Design review of the part built by this model. Coordinates are the model's own, in mm. A direction names the side the tool comes from. Coordinates: 2 decimals unless noted, no trailing zeros. Order: outer loops, then holes, each group sorted by start corner. A loop starts at its lowest first (then second) coordinate and runs counter-clockwise, first axis right, second up. Notation, with made-up numbers: (52, 64.5) - (59, 64.5) arc R12 ccw to (59, 78.5) - close; hole circle Ø10 at (-14, -39). An arc over 180 degrees is marked (long way). Write each question's results on one line, items separated by ' | '. Start each with the question number.
```python
from build123d import *

# Parameters (mm, degrees)
SKETCH1_W                                       = 146
SKETCH1_H                                       = 85
BOSS_EXTRUDE1_DEPTH                             = 15
SHELL1_T                                        = -5
SKETCH2_W                                       = 5
SKETCH2_H                                       = 75
CUT_EXTRUDE1_DEPTH                              = 10
BOSS_EXTRUDE2_DEPTH                             = 10
CSK_FOR_M3_FLAT_HEAD_MACHINE_SCREW1_D           = 3.4
CSK_FOR_M3_FLAT_HEAD_MACHINE_SCREW1_DEPTH       = 10
CSK_FOR_M3_FLAT_HEAD_MACHINE_SCREW1_CSINK_D     = 6.3
CSK_FOR_M3_FLAT_HEAD_MACHINE_SCREW1_CSINK_ANGLE = 90
CSK_FOR_M3_FLAT_HEAD_MACHINE_SCREW1_TIP         = 1.021463052
FILLET1_R                                       = 3
CUT_EXTRUDE3_DEPTH                              = 10
FILLET2_R                                       = 2
SKETCH13_W                                      = 12
SKETCH13_H                                      = 8
CUT_EXTRUDE5_DEPTH                              = 86.791899384
FILLET3_R                                       = 2
SKETCH14_R                                      = 5
BOSS_EXTRUDE4_DEPTH                             = 5
F_4_0_4_DIAMETER_HOLE2_D                        = 4
CUT_EXTRUDE6_DEPTH                              = 2
SKETCH19_W                                      = 61
SKETCH19_H                                      = 36
CUT_EXTRUDE7_DEPTH                              = 1


with BuildPart() as part:
    # Sketch1 → Boss-Extrude1 (new body)
    with BuildSketch(Plane(origin=(0, 0, 0), x_dir=(1, 0, 0), z_dir=(0, 1, 0))):
        Rectangle(SKETCH1_W, SKETCH1_H)
    extrude(amount=BOSS_EXTRUDE1_DEPTH)

    # Shell1
    shell1_openings = [part.faces().sort_by_distance(p)[0] for p in [
        (0, 15, 0),
    ]]
    offset(amount=SHELL1_T, openings=shell1_openings, kind=Kind.INTERSECTION)

    # Sketch2 → Cut-Extrude1 (cut)
    with BuildSketch(Plane(origin=(0, 15, 0), x_dir=(1, 0, 0), z_dir=(0, 1, 0))):
        with Locations((-70.5, 0)):
            Rectangle(SKETCH2_W, SKETCH2_H)
    extrude(amount=-CUT_EXTRUDE1_DEPTH, mode=Mode.SUBTRACT)

    # Sketch3 → Boss-Extrude2 (add)
    with BuildSketch(Plane(origin=(0, 5, 0), x_dir=(1, 0, 0), z_dir=(0, 1, 0))):
        Polygon((-55.5, 30.5), (50.5, 30.5), (57.5, 37.5), (-62.5, 37.5), align=None)
        Polygon((-55.5, -30.5), (-62.5, -37.5), (57.5, -37.5), (50.5, -30.5), align=None)
    extrude(amount=BOSS_EXTRUDE2_DEPTH)

    # CSK for M3 Flat Head Machine Screw1
    with Locations(Plane(origin=(0, 0, 0), x_dir=(-1, 0, 0), z_dir=(0, -1, 0))):
        with Locations((-63, -33), (67, 33), (67, -33), (-63, 33)):
            CounterSinkHole(CSK_FOR_M3_FLAT_HEAD_MACHINE_SCREW1_D / 2, CSK_FOR_M3_FLAT_HEAD_MACHINE_SCREW1_CSINK_D / 2, depth=CSK_FOR_M3_FLAT_HEAD_MACHINE_SCREW1_DEPTH, counter_sink_angle=CSK_FOR_M3_FLAT_HEAD_MACHINE_SCREW1_CSINK_ANGLE)
            with Locations((0, 0, -(CSK_FOR_M3_FLAT_HEAD_MACHINE_SCREW1_DEPTH + CSK_FOR_M3_FLAT_HEAD_MACHINE_SCREW1_TIP / 2))):  # 118° drill point
                Cone(0, CSK_FOR_M3_FLAT_HEAD_MACHINE_SCREW1_D / 2, CSK_FOR_M3_FLAT_HEAD_MACHINE_SCREW1_TIP, mode=Mode.SUBTRACT)

    # Fillet1
    fillet1_edges = [part.edges().sort_by_distance(p)[0] for p in [
        (-73, 7.5, -42.5),
        (73, 7.5, -42.5),
        (73, 7.5, 42.5),
        (-73, 7.5, 42.5),
    ]]
    fillet(fillet1_edges, radius=FILLET1_R)

    # Sketch8 → Cut-Extrude3 (cut)
    with BuildSketch(Plane.XZ):
        Polygon((67.5, 0), (37.5, 29), (37.5, -29), align=None)
        Polygon((0, 4.537548682), (25.305984122, 29), (-25.305984122, 29), align=None)
        Polygon((2.5, 0), (32.5, -29), (32.5, 29), align=None)
        Polygon((-2.5, 0), (-32.5, 29), (-32.5, -29), align=None)
        Polygon((-67.5, 0), (-37.5, -29), (-37.5, 29), align=None)
        Polygon((-44.694015878, 29), (-67.5, 29), (-67.5, 6.954215348), align=None)
        Polygon((67.5, 6.954215348), (44.694015878, 29), (67.5, 29), align=None)
        Polygon((44.694015878, -29), (67.5, -29), (67.5, -6.954215348), align=None)
        Polygon((-67.5, -6.954215348), (-44.694015878, -29), (-67.5, -29), align=None)
        Polygon((-25.305984122, -29), (25.305984122, -29), (0, -4.537548682), align=None)
    extrude(amount=-CUT_EXTRUDE3_DEPTH, mode=Mode.SUBTRACT)

    # Fillet2
    fillet2_edges = [part.edges().sort_by_distance(p)[0] for p in [
        (-67.5, 2.5, 0),
        (-37.5, 2.5, 29),
        (-37.5, 2.5, -29),
        (0, 2.5, 4.537548682),
        (-25.305984122, 2.5, 29),
        (25.305984122, 2.5, 29),
        (44.694015878, 2.5, -29),
        (67.5, 2.5, -6.954215348),
        (67.5, 2.5, -29),
        (-67.5, 2.5, -29),
        (-67.5, 2.5, -6.954215348),
        (-44.694015878, 2.5, -29),
        (67.5, 2.5, 29),
        (67.5, 2.5, 6.954215348),
        (44.694015878, 2.5, 29),
        (-44.694015878, 2.5, 29),
        (-67.5, 2.5, 6.954215348),
        (-67.5, 2.5, 29),
        (-2.5, 2.5, 0),
        (-32.5, 2.5, -29),
        (-32.5, 2.5, 29),
        (2.5, 2.5, 0),
        (32.5, 2.5, 29),
        (32.5, 2.5, -29),
        (-25.305984122, 2.5, -29),
        (0, 2.5, -4.537548682),
        (25.305984122, 2.5, -29),
        (67.5, 2.5, 0),
        (37.5, 2.5, -29),
        (37.5, 2.5, 29),
    ]]
    fillet(fillet2_edges, radius=FILLET2_R)

    # Sketch13 → Cut-Extrude5 (cut, through all)
    with BuildSketch(Plane.XZ):
        with Locations((-35, -36.5)):
            Rectangle(SKETCH13_W, SKETCH13_H)
    extrude(amount=-CUT_EXTRUDE5_DEPTH, mode=Mode.SUBTRACT)

    # Fillet3
    fillet3_edges = [part.edges().sort_by_distance(p)[0] for p in [
        (-41, 7.5, -40.5),
        (-41, 7.5, -32.5),
        (-29, 7.5, -32.5),
        (-29, 7.5, -40.5),
    ]]
    fillet(fillet3_edges, radius=FILLET3_R)

    # Sketch14 → Boss-Extrude4 (add, through all)
    with BuildSketch(Plane(origin=(0, 5, 0), x_dir=(1, 0, 0), z_dir=(0, 1, 0))):
        with Locations((-35, 0)):
            Circle(SKETCH14_R)
    extrude(amount=-BOSS_EXTRUDE4_DEPTH)

    # Ø4.0 (4) Diameter Hole2 (through all)
    with Locations(Plane(origin=(0, 5, 0), x_dir=(1, 0, 0), z_dir=(0, 1, 0))):
        with Locations((-35, 0)):
            Hole(F_4_0_4_DIAMETER_HOLE2_D / 2)

    # Sketch17 → Cut-Extrude6 (cut)
    with BuildSketch(Plane(origin=(0, 5, 0), x_dir=(1, 0, 0), z_dir=(0, 1, 0))):
        Polygon((-31.766838493, 0), (-33.383419246, 2.8), (-36.616580754, 2.8), (-38.233161507, 0), (-36.616580754, -2.8), (-33.383419246, -2.8), align=None)
    extrude(amount=-CUT_EXTRUDE6_DEPTH, mode=Mode.SUBTRACT)

    # Sketch19 → Cut-Extrude7 (cut)
    with BuildSketch(Plane.XZ):
        with Locations((-35, 0)):
            Rectangle(SKETCH19_W, SKETCH19_H)
    extrude(amount=-CUT_EXTRUDE7_DEPTH, mode=Mode.SUBTRACT)


solid = part.part
```
(1) Mouldability with a two-part tool opening along X and no side actions: class faces 3 (the face through (-2, 10, 30.5)), 4 (the face through (-31.311, 2.535, 26.113)) as +X half, -X half, draft (parallel to the pull), parting line (faces both ways), or undercut.
(2) Take a section at A-A (z = 33). State the section outline as (x, y) points.
(3) Take a section at D-D (z = -16). State how many separate pieces and enclosed holes the cut face has, plus the area to 3 significant figures.
(4) Clearance check with flat-ended pins moving along their axes: pin 1 (5 mm diameter, centred on y = 10, z = -15.5, fed in from -X); pin 2 (5 mm diameter, centred on x = -35, z = 0, fed in from +Y); pin 3 (5 mm diameter, centred on x = -12, z = -8, fed in from -Y). State where each tip first meets the part, or that it passes through.
(5) Tool access review of faces 1 (the face through (-32.8, 1, 0.3)), 2 (the face through (-35, 7, -40.5)): name each direction out of +Z, -Z, +X, -X, +Y, -Y from which nothing blocks a thin tool from reaching the whole face with its end or side.
(6) Take a section at B-B (x = -35). State the section outline as (y, z) points.
(7) Take a section at C-C (y = 13). State the section outline as (x, z) points, plus the area to 3 significant figures.
(8) To check wall thickness, follow line 1 along X through (y, z) = (3.05, 33); line 2 along Z through (x, y) = (48, 12.5); line 3 along Z through (x, y) = (-62.5, 5.75). State the ranges of each line that lie inside material, in increasing order. Write a range as [from, to].
Worked out:
1) face 3: draft | face 4: undercut
2) outline: (-73, 0) - (-70.15, 0) - (-68.7, 1.45) - (-68.7, 5) - (-73, 5) - close; (-65.3, 1.45) - (-63.85, 0) - (59.85, 0) - (61.3, 1.45) - (61.3, 5) - (53, 5) - (53, 15) - (-58, 15) - (-58, 5) - (-65.3, 5) - close; (64.7, 1.45) - (66.15, 0) - (73, 0) - (73, 15) - (68, 15) - (68, 5) - (64.7, 5) - close
3) separate pieces: 8 | enclosed holes: 0 | area: 279 mm^2
4) pin 1: x = 68 | pin 2: y = 3 | pin 3: y = 1
5) face 1: -Y | face 2: +Y, -Y
6) outline: (0, -42.5) - (15, -42.5) - (15, -40.5) - (0, -40.5) - close; (0, -32.5) - (15, -32.5) - (15, -30.5) - (5, -30.5) - (5, -2.8) - (3, -2.8) - (3, -2) - (1, -2) - (1, -18) - (0, -18) - close; (0, 18) - (1, 18) - (1, 2) - (3, 2) - (3, 2.8) - (5, 2.8) - (5, 30.5) - (15, 30.5) - (15, 42.5) - (0, 42.5) - close
7) outline: (-73, -39.5) arc R3 ccw to (-70, -42.5) - (70, -42.5) arc R3 ccw to (73, -39.5) - (73, 39.5) arc R3 ccw to (70, 42.5) - (-70, 42.5) arc R3 ccw to (-73, 39.5) - (-73, 37.5) - (-62.5, 37.5) - (-55.5, 30.5) - (50.5, 30.5) - (57.5, 37.5) - (68, 37.5) - (68, -37.5) - (57.5, -37.5) - (50.5, -30.5) - (-55.5, -30.5) - (-62.5, -37.5) - (-73, -37.5) - close; hole (-41, -38.5) arc R2 ccw to (-39, -40.5) - (-31, -40.5) arc R2 ccw to (-29, -38.5) - (-29, -34.5) arc R2 ccw to (-31, -32.5) - (-39, -32.5) arc R2 ccw to (-41, -34.5) - close | area: 3,320 mm^2
8) line 1: [-73, -68.7], [-65.3, 61.3], [64.7, 73] | line 2: [-42.5, -30.5], [30.5, 42.5] | line 3: [-42.5, -37.5], [37.5, 42.5]
